from build123d import *

# Parameters (mm, degrees)
F1_DEPTH     = 5
F2_R         = 8.75
F2_R_2       = 18.75
F2_R_3       = 26.25
F3_DEPTH     = 2
F5_DEPTH     = 12
F6_R         = 3.175
F7_DEPTH     = 183.6597451804
F8_R         = 5.08
F9_DEPTH     = 30
F10_S5_R     = 5.08
F10_T6_DEPTH = 9
F11_R        = 10


# Not quite as in the source:
# - a fillet or chamfer that OpenCascade refuses, or shapes differently, is made with other operations: its cross-section is extruded or revolved along the edge and cut away or added


with BuildPart() as f1:
    # F0 (on Top) → F1 (new body)
    with BuildSketch(Plane.XY):
        with BuildLine():
            ThreePointArc((89.2893218813, 160), (59.2982241526, 155.6212032378), (31.8110246399, 142.8503901468))
            ThreePointArc((31.8110246399, 142.8503901468), (29.1326558006, 125.6088436513), (46.5579786953, 124.7129043596))
            ThreePointArc((46.5579786953, 124.7129043596), (54.6897066789, 124.7129043596), (54.6897066789, 116.581176376))
            ThreePointArc((54.6897066789, 116.581176376), (54.6897066789, 85.8220313944), (85.4488516605, 85.8220313944))
            ThreePointArc((85.4488516605, 85.8220313944), (98.8838805031, 85.8220313944), (98.8838805031, 72.3870025518))
            ThreePointArc((98.8838805031, 72.3870025518), (101.1313528665, 28.995133397), (144.0588384666, 35.7134978428))
            ThreePointArc((144.0588384666, 35.7134978428), (155.9302038799, 61.3407550467), (160, 89.2893218813))
            Line((160, 89.2893218813), (160, 148.686291501))
            Line((160, 148.686291501), (148.686291501, 160))
            Line((148.686291501, 160), (89.2893218813, 160))
        make_face()
    extrude(amount=-F1_DEPTH)

    # F2 (on Top) → F3 (cut)
    with BuildSketch(Plane.XY):
        with Locations((38.2494740163, 133.0214090386)):
            Circle(F2_R)
        with Locations((70.0692791697, 101.2016038852)):
            Circle(F2_R_2)
        with Locations((119.5667538528, 51.7041292021)):
            Circle(F2_R_3)
    extrude(amount=-F3_DEPTH, mode=Mode.SUBTRACT)

    # F4 (on Top) → F5 (join)
    with BuildSketch(Plane.XY):
        Polygon((160, 148.686291501), (148.686291501, 160), (89.2893218813, 160), (160, 89.2893218813), align=None)
    extrude(amount=F5_DEPTH)

    # F6 (on face) → F7 (cut, through all)
    with BuildSketch(Plane(origin=(154.3431457505, 154.3431457505, 0), x_dir=(-0.7071067812, 0.7071067812, 0), z_dir=(0.7071067812, 0.7071067812, 0))):
        with Locations((0, 5.08)):
            Circle(F6_R)
    extrude(amount=-F7_DEPTH, mode=Mode.SUBTRACT)

    # F8 (on face) → F9 (cut)
    with BuildSketch(Plane(origin=(124.6446609407, 124.6446609407, 0), x_dir=(0.7071067812, -0.7071067812, 0), z_dir=(-0.7071067812, -0.7071067812, 0))):
        with Locations((0, 5.08)):
            Circle(F8_R)
    extrude(amount=-F9_DEPTH, mode=Mode.SUBTRACT)

    # F10: chamfer of 2 on 1 edges, made by hand


with BuildPart() as f10_tool2:
    # F10_s3 → F10_t4 (revolve)
    with BuildSketch(Plane.XY.offset(5.08)):
        Polygon((145.0270139084, 149.5171419689), (142.1985867836, 149.5171419689), (143.612800346, 148.1029284065), align=None)
    revolve(axis=Axis((145.8578643763, 145.8578643763, 5.08), (0.7071067812, 0.7071067812, 0)))

    # F10_s5 → F10_t6 (intersect, symmetric)
    with BuildSketch(Plane(origin=(145.8761289588, 145.8761289588, 0), x_dir=(0, 0, 1), z_dir=(-0.7071067812, -0.7071067812, 0))):
        with Locations((5.08, 0)):
            Circle(F10_S5_R)
    extrude(amount=F10_T6_DEPTH, both=True, mode=Mode.INTERSECT)


with BuildPart() as f1_1:
    add(f1.part)

    # F10_t1: cut F10_tool2
    add(f10_tool2.part, mode=Mode.SUBTRACT)

    # F11
    f11_edges = [f1_1.edges().sort_by_distance(p)[0] for p in [
        (160, 89.289322, 6),
        (89.289322, 160, 6),
    ]]
    fillet(f11_edges, radius=F11_R)


solid = f1_1.part
Model file for the job. Use its own axes, mm. A direction names the side the tool comes from. Give positions to 0.01 mm unless a question says otherwise; leave off trailing zeros. Order: outer loops, then holes, each group sorted by start corner. A loop starts at its lowest first (then second) coordinate and runs counter-clockwise, first axis right, second up. Notation, with made-up numbers: (87.25, 6.5) - (96.25, 6.5) arc R8 cw to (96.25, 19.5) - close; hole circle Ø2 at (49, 24). An arc over 180 degrees is marked (long way). Write item = value, one per line. Start each with the question number.
1. Drop flat-ended pins along their axis: P1, Ø20, axis at x = 38.25, y = 133.02, coming from the +Z side; P2, Ø10, axis at y = 103, z = 7, coming from the -X side; P3, Ø6, axis at x = 118.5, z = 5, coming from the -Y side. Give the stop position or say it passes through.
2. Probe line 1 along Y through (x, z) = (143, 1); line 2 along X through (y, z) = (69, -1.25); line 3 along Z through (x, y) = (52, 128.5). List the from-to ranges inside material, lowest first.
3. Two-plate mould, pull along X, no slides. Class faces 5 (the flat face through (154.422, 154.264, 1.492)), 6 (the cylindrical face through (138.47, 131.8, 6.97)), 7 (the flat face through (107, 107, -5)): pulls with the +X half, pulls with the -X half, needs draft (parallel to the pull), parting line crosses it, or undercut.
4. Which spindle directions (+Z, -Z, +X, -X, +Y, -Y) get a long thin tool onto all of the face, cutting with end or side? Do faces 1 (the conical face through (149.04, 145.34, 3.08)), 2 (the cylindrical face through (104.257, 153.979, 6.084)), 3 (the flat face through (119, 52, -2)), 4 (the flat face through (124.39, 124.9, 11.25)). Say none if no direction does.
5. Cut at A-A, the plane y = 60. List the corners of the cut face in (x, z).
6. Cut at B-B, the plane x = 43. List the corners of the cut face in (y, z), and give its area (3 significant figures).
Taken from the geometry:
q1.P1 = 0
q1.P2 = 141.29
q1.P3 = 128.1
q2.line_1 = 106.29 to 138.72, 147.28 to 160
q2.line_2 = 95.98 to 99.82, 139.31 to 157.88
q2.line_3 = -5 to 0
q3.face_5 = pulls with the +X half
q3.face_6 = undercut
q3.face_7 = needs draft
q4.face_1 = none
q4.face_2 = +Z, -X
q4.face_3 = +Z
q4.face_4 = +Z, -X, -Y
q5.outline = (91.52, -5) - (155.52, -5) - (155.52, 0) - (144.47, 0) - (144.47, -2) - (94.66, -2) - (94.66, 0) - (91.52, 0) - close
q6.outline = (122.27, -5) - (149.23, -5) - (149.23, 0) - (140.37, 0) - (140.37, -2) - (125.67, -2) - (125.67, 0) - (122.27, 0) - close
q6.area = 105 mm²
